Geometry check sheet. Reference: the model listing, model coordinates, mm. Round coordinates to 2 decimals unless told otherwise and drop trailing zeros. Order: outer loops, then holes, each group sorted by start corner. A loop starts at its lowest first (then second) coordinate and runs counter-clockwise, first axis right, second up.
(1) Sectioned sample at A-A (z = -48). Record the boundary of the cut face in (x, y).
(2) Material ranges on line 1 along X through (y, z) = (0.7, 5); line 2 along X through (y, z) = (0.7, 47.5), recorded low to high.
(3) Go/stop test with a flat-tipped pin: pin 1 (3.5 mm diameter, centred on x = -82, z = -5, fed in from +Y). Record where the tip stops, or that it passes through.
(4) Sectioned sample at C-C (y = 0.5). Give the number of separate pieces and of enclosed holes in the cut face, plus the area to 3 significant figures.
(5) Sectioned sample at B-B (x = 51.5). Record the boundary of the cut face in (y, z).
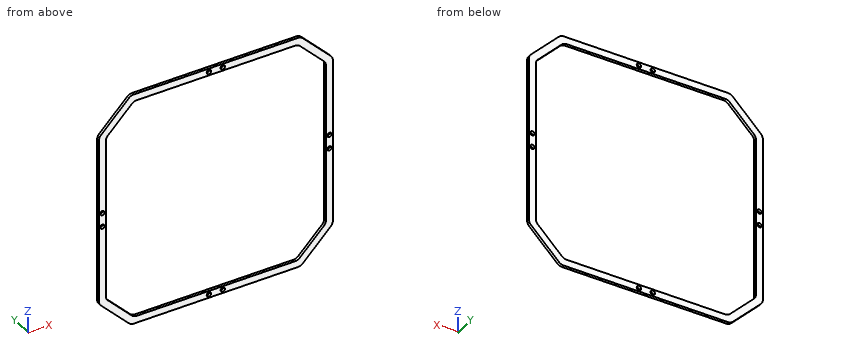
from build123d import *

# Parameters (mm, degrees)
SKETCH_1_R      = 1.6
EXTRUDE_1_DEPTH = 2


with BuildPart() as part:
    # 草图1 → 凸台-拉伸1 (new body)
    with BuildSketch(Plane(origin=(0, 0, 0), x_dir=(1, 0, 0), z_dir=(0, 1, 0))):
        with BuildLine():
            Line((0, 84.5), (59.290367902, 84.5))
            ThreePointArc((59.290367902, 84.5), (61.203785064, 84.119397663), (62.825901808, 83.035533906))
            Line((62.825901808, 83.035533906), (83.035533906, 62.825901808))
            ThreePointArc((83.035533906, 62.825901808), (84.119397663, 61.203785064), (84.5, 59.290367902))
            Line((84.5, 59.290367902), (84.5, 0))
            Line((84.5, 0), (84.5, -59.290367902))
            ThreePointArc((84.5, -59.290367902), (84.119397663, -61.203785064), (83.035533906, -62.825901808))
            Line((83.035533906, -62.825901808), (62.825901808, -83.035533906))
            ThreePointArc((62.825901808, -83.035533906), (61.203785064, -84.119397663), (59.290367902, -84.5))
            Line((59.290367902, -84.5), (0, -84.5))
            Line((0, -84.5), (-59.290367902, -84.5))
            ThreePointArc((-59.290367902, -84.5), (-61.203785064, -84.119397663), (-62.825901808, -83.035533906))
            Line((-62.825901808, -83.035533906), (-83.035533906, -62.825901808))
            ThreePointArc((-83.035533906, -62.825901808), (-84.119397663, -61.203785064), (-84.5, -59.290367902))
            Line((-84.5, -59.290367902), (-84.5, -1.780508218))
            Line((-84.5, -1.780508218), (-84.5, 59.290367902))
            ThreePointArc((-84.5, 59.290367902), (-84.119397663, 61.203785064), (-83.035533906, 62.825901808))
            Line((-83.035533906, 62.825901808), (-62.825901808, 83.035533906))
            ThreePointArc((-62.825901808, 83.035533906), (-61.203785064, 84.119397663), (-59.290367902, 84.5))
            Line((-59.290367902, 84.5), (0, 84.5))
        make_face()
        with Locations(Location((5, 82, 0), (0, 0, 270))):
            Circle(SKETCH_1_R, mode=Mode.SUBTRACT)
        with Locations(Location((-5, 82, 0), (0, 0, 270))):
            Circle(SKETCH_1_R, mode=Mode.SUBTRACT)
        with Locations(Location((82, 5, 0), (0, 0, 270))):
            Circle(SKETCH_1_R, mode=Mode.SUBTRACT)
        with Locations(Location((82, -5, 0), (0, 0, 270))):
            Circle(SKETCH_1_R, mode=Mode.SUBTRACT)
        with Locations(Location((5, -82, 0), (0, 0, 270))):
            Circle(SKETCH_1_R, mode=Mode.SUBTRACT)
        with Locations(Location((-5, -82, 0), (0, 0, 270))):
            Circle(SKETCH_1_R, mode=Mode.SUBTRACT)
        with Locations(Location((-82, -5, 0), (0, 0, 270))):
            Circle(SKETCH_1_R, mode=Mode.SUBTRACT)
        with Locations(Location((-82, 5, 0), (0, 0, 270))):
            Circle(SKETCH_1_R, mode=Mode.SUBTRACT)
        with BuildLine():
            Line((0, 79.5), (57.21930009, 79.5))
            ThreePointArc((57.21930009, 79.5), (59.132717252, 79.119397663), (60.754833996, 78.035533906))
            Line((60.754833996, 78.035533906), (78.035533906, 60.754833996))
            ThreePointArc((78.035533906, 60.754833996), (79.119397663, 59.132717252), (79.5, 57.21930009))
            Line((79.5, 57.21930009), (79.5, 0))
            Line((79.5, 0), (79.5, -57.21930009))
            ThreePointArc((79.5, -57.21930009), (79.119397663, -59.132717252), (78.035533906, -60.754833996))
            Line((78.035533906, -60.754833996), (60.754833996, -78.035533906))
            ThreePointArc((60.754833996, -78.035533906), (59.132717252, -79.119397663), (57.21930009, -79.5))
            Line((57.21930009, -79.5), (0, -79.5))
            Line((0, -79.5), (-57.21930009, -79.5))
            ThreePointArc((-57.21930009, -79.5), (-59.132717252, -79.119397663), (-60.754833996, -78.035533906))
            Line((-60.754833996, -78.035533906), (-78.035533906, -60.754833996))
            ThreePointArc((-78.035533906, -60.754833996), (-79.119397663, -59.132717252), (-79.5, -57.21930009))
            Line((-79.5, -57.21930009), (-79.5, -1.165353087))
            Line((-79.5, -1.165353087), (-79.5, 57.21930009))
            ThreePointArc((-79.5, 57.21930009), (-79.119397663, 59.132717252), (-78.035533906, 60.754833996))
            Line((-78.035533906, 60.754833996), (-60.754833996, 78.035533906))
            ThreePointArc((-60.754833996, 78.035533906), (-59.132717252, 79.119397663), (-57.21930009, 79.5))
            Line((-57.21930009, 79.5), (0, 79.5))
        make_face(mode=Mode.SUBTRACT)
    extrude(amount=EXTRUDE_1_DEPTH)


solid = part.part
Answer below:
1. outline: (-84.5, 0) - (-79.5, 0) - (-79.5, 2) - (-84.5, 2) - close; (79.5, 0) - (84.5, 0) - (84.5, 2) - (79.5, 2) - close
2. line 1: x = -84.5 to -83.6, -80.4 to -79.5, 79.5 to 80.4, 83.6 to 84.5
2. line 2: x = -84.5 to -79.5, 79.5 to 84.5
3. pin 1: stops at y = 2
4. separate pieces: 1
4. enclosed holes: 9
4. area: 2,960 mm2
5. outline: (0, -84.5) - (2, -84.5) - (2, -79.5) - (0, -79.5) - close; (0, 79.5) - (2, 79.5) - (2, 84.5) - (0, 84.5) - close
